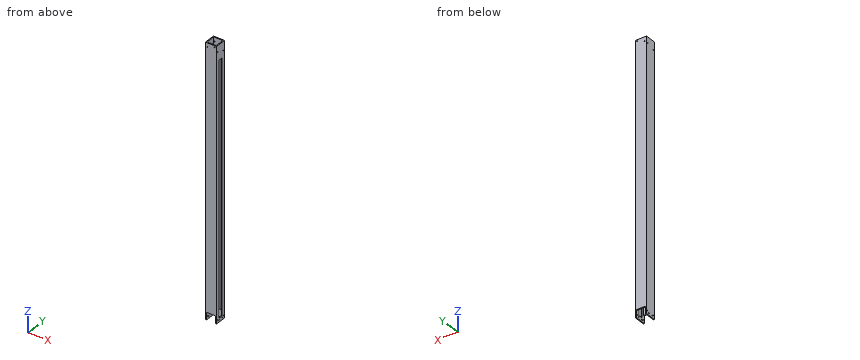
from build123d import *

# Parameters (mm, degrees)
BOSS_EXTRUDE1_DEPTH     = 914.4
CUT_EXTRUDE2_DEPTH      = 70.104
CUT_EXTRUDE2_DEPTH_BACK = 58.42
SKETCH7_R               = 1.75
SKETCH8_W               = 31.4325
SKETCH8_H               = 50.8
CUT_EXTRUDE3_DEPTH      = 71.882
SKETCH10_R              = 1.75
CUT_EXTRUDE5_DEPTH      = 12.7
SKETCH11_W              = 13.97
SKETCH11_H              = 12.7
BOSS_EXTRUDE2_DEPTH     = 3.33375
SKETCH9_R               = 1.75
CUT_EXTRUDE4_DEPTH      = 68.326
CIRPATTERN1_COUNT       = 2
SKETCH12_W              = 38.1
SKETCH12_H              = 50.8
SKETCH12_R              = 1.75
BOSS_EXTRUDE3_DEPTH     = 3.33375


with BuildPart() as part:
    # Sketch1 → Boss-Extrude1 (new body)
    with BuildSketch(Plane(origin=(0, 0, 0), x_dir=(0, 1, 0), z_dir=(0, 0, 1))):
        Polygon((6.985, -19.05), (19.05, -19.05), (19.05, 19.05), (-19.05, 19.05), (-19.05, -19.05), (-6.985, -19.05), (-6.985, -15.71625), (-15.71625, -15.71625), (-15.71625, 15.71625), (15.71625, 15.71625), (15.71625, -15.71625), (6.985, -15.71625), align=None)
    extrude(amount=BOSS_EXTRUDE1_DEPTH)

    # Sketch7 → Cut-Extrude2 (cut, two sides: drawn at the far end of the back side and taken through both)
    with BuildSketch(Plane(origin=(0, 0, 0), x_dir=(-1, 0, 0), z_dir=(0, 1, 0)).offset(-CUT_EXTRUDE2_DEPTH_BACK)):
        with Locations(Location((-12.7, 909.6375, 0), (0, 0, 270))):
            Circle(SKETCH7_R)
        with Locations(Location((12.7, 900.1125, 0), (0, 0, 270))):
            Circle(SKETCH7_R)
    extrude(amount=CUT_EXTRUDE2_DEPTH + CUT_EXTRUDE2_DEPTH_BACK, mode=Mode.SUBTRACT)

    # Sketch8 → Cut-Extrude3 (cut)
    with BuildSketch(Plane(origin=(0, 19.05, 0), x_dir=(-1, 0, 0), z_dir=(0, 1, 0))):
        Rectangle(SKETCH8_W, SKETCH8_H)
    extrude(amount=-CUT_EXTRUDE3_DEPTH, mode=Mode.SUBTRACT)

    # Sketch10 → Cut-Extrude5 (cut)
    with BuildSketch(Plane.YZ.offset(19.05)):
        with Locations((-12.7, 893.7625)):
            Circle(SKETCH10_R)
        with Locations((12.7, 884.2375)):
            Circle(SKETCH10_R)
    cut_extrude5 = extrude(amount=-CUT_EXTRUDE5_DEPTH, mode=Mode.SUBTRACT)

    # Sketch11 → Boss-Extrude2 (add)
    with BuildSketch(Plane.YZ.offset(19.05)):
        with Locations((0, 6.35)):
            Rectangle(SKETCH11_W, SKETCH11_H)
    extrude(amount=-BOSS_EXTRUDE2_DEPTH)

    # Sketch9 → Cut-Extrude4 (cut)
    with BuildSketch(Plane.YZ.offset(19.05)):
        with Locations((-15.24, 10.795)):
            Circle(SKETCH9_R)
        with Locations((15.24, 10.795)):
            Circle(SKETCH9_R)
        with Locations((7.62, 6.985)):
            Circle(SKETCH9_R)
        with Locations((-7.62, 6.985)):
            Circle(SKETCH9_R)
    extrude(amount=-CUT_EXTRUDE4_DEPTH, mode=Mode.SUBTRACT)

    # CirPattern1: Cut-Extrude5 ×2 about axis
    cirpattern1_axis = Axis((0, 0, 746.76), (0, 0, -1))
    for i in range(1, CIRPATTERN1_COUNT):
        add(cut_extrude5.rotate(cirpattern1_axis, i * 360 / CIRPATTERN1_COUNT), mode=Mode.SUBTRACT)

    # Sketch12 → Boss-Extrude3 (add)
    with BuildSketch(Plane.YZ.offset(19.05)):
        with Locations((0, 889)):
            Rectangle(SKETCH12_W, SKETCH12_H)
        with Locations((12.7, 884.2375)):
            Circle(SKETCH12_R, mode=Mode.SUBTRACT)
        with Locations((-12.7, 893.7625)):
            Circle(SKETCH12_R, mode=Mode.SUBTRACT)
    extrude(amount=-BOSS_EXTRUDE3_DEPTH)


solid = part.part
Model file for the job. Use its own axes, mm. Give positions to 0.01 mm unless a question says otherwise; leave off trailing zeros. Order: outer loops, then holes, each group sorted by start corner. A loop starts at its lowest first (then second) coordinate and runs counter-clockwise, first axis right, second up. Notation, with made-up numbers: M 3,10 L 10,10 A16 cw 10,34 Z; hole C 50,53 d4. An arc over 180 degrees is marked long. Write item = value, one per line.
Q1. Cut at A-A, the plane y = 0. List the corners of the cut face in (x, z), then the cut area to 3 significant figures.
Derived:
outline = M -19.05,0 L -15.72,0 L -15.72,914.4 L -19.05,914.4 Z; M 15.72,0 L 19.05,0 L 19.05,12.7 L 15.72,12.7 Z; M 15.72,863.6 L 19.05,863.6 L 19.05,914.4 L 15.72,914.4 Z
area = 3,260 mm2
Q2. Flat gauge pins, fed straight in: pin 1 (3.5 mm diameter, centred on x = -6.5, y = 17, fed in from -Z); pin 2 (3 mm diameter, centred on y = -12.7, z = 893.76, fed in from +X); pin 3 (3 mm diameter, centred on x = 12.7, z = 909.64, fed in from -Y). Where does each tip first touch, or does it go through?
Derived:
pin_1 = 25.4
pin_2 = -15.72
pin_3 = through
Q3. Cut at B-B, the plane z = 421.5. List the corners of the cut face in (x, y) (3 decimals), then the cut area to 3 significant figures.
Derived:
outline = M -19.05,-19.05 L 19.05,-19.05 L 19.05,-6.985 L 15.716,-6.985 L 15.716,-15.716 L -15.716,-15.716 L -15.716,15.716 L 15.716,15.716 L 15.716,6.985 L 19.05,6.985 L 19.05,19.05 L -19.05,19.05 Z
area = 417 mm2
Q4. Drill centre lines: line 1 (X direction, y = 1, z = 865.5); line 2 (Z direction, x = -16.7, y = 12.7). Where is each one in solid material? Low to high. Write a range as [from, to].
Derived:
line_1 = [-19.05, -15.72], [15.72, 19.05]
line_2 = [0, 892.01], [895.51, 914.4]
